Can you work these out from the model? Positions are in its coordinate system, mm. A direction names the side the tool comes from. Give positions to 0.01 mm unless a question says otherwise; leave off trailing zeros. Loops run counter-clockwise (first coordinate to the right, second up) from the corner with the lowest first, then second, coordinate; pieces in that order, holes last.
from build123d import *

# Parameters (mm, degrees)
SKETCH1_R           = 1.75
BOSS_EXTRUDE1_DEPTH = 5
SKETCH3_W           = 35
SKETCH3_H           = 20
SKETCH3_W_2         = 22.6
SKETCH3_H_2         = 12
BOSS_EXTRUDE4_DEPTH = 3
SKETCH6_W           = 15.399861764
SKETCH6_H           = 20
CUT_EXTRUDE2_DEPTH  = 76.166481892
SKETCH9_R           = 1
CUT_EXTRUDE4_DEPTH  = 7
SKETCH24_W          = 38
SKETCH24_H          = 25
BOSS_EXTRUDE8_DEPTH = 5
SKETCH27_R          = 2.3
CUT_EXTRUDE15_DEPTH = 4
FILLET9_R           = 4
SKETCH3_5_W         = 22.6
SKETCH3_5_H         = 12
CUT_EXTRUDE16_DEPTH = 3
BOSS_EXTRUDE9_DEPTH = 2
CUT_EXTRUDE18_DEPTH = 4
CUT_EXTRUDE19_DEPTH = 66.796921133
SKETCH37_W          = 38
SKETCH37_H          = 4.5
CUT_EXTRUDE20_DEPTH = 4


with BuildPart() as part:
    # Sketch1 → Boss-Extrude1 (new body)
    with BuildSketch(Plane(origin=(0, 0, 0), x_dir=(1, 0, 0), z_dir=(0, 1, 0))):
        Polygon((0, 33.819660113), (0, 15), (10, 0), (26, 0), (36, 15), (60, 15), (60, 35), (36, 35), (26, 45), (10, 45), align=None)
        with Locations(Location((13, 5, 0), (0, 0, 270))):
            Circle(SKETCH1_R, mode=Mode.SUBTRACT)
        with Locations(Location((23, 5, 0), (0, 0, 270))):
            Circle(SKETCH1_R, mode=Mode.SUBTRACT)
        with Locations(Location((5, 25, 0), (0, 0, 270))):
            Circle(SKETCH1_R, mode=Mode.SUBTRACT)
    extrude(amount=BOSS_EXTRUDE1_DEPTH)

    # Sketch3 → Boss-Extrude4 (add)
    with BuildSketch(Plane.XZ):
        with Locations((27.100138236, -25)):
            Rectangle(SKETCH3_W, SKETCH3_H)
        with Locations((27.100138236, -25)):
            Rectangle(SKETCH3_W_2, SKETCH3_H_2, mode=Mode.SUBTRACT)
    extrude(amount=BOSS_EXTRUDE4_DEPTH)

    # Sketch6 → Cut-Extrude2 (cut, through all)
    with BuildSketch(Plane.XZ):
        with Locations((52.300069118, -25)):
            Rectangle(SKETCH6_W, SKETCH6_H)
    extrude(amount=-CUT_EXTRUDE2_DEPTH, mode=Mode.SUBTRACT)

    # Sketch9 → Cut-Extrude4 (cut)
    with BuildSketch(Plane.XZ.offset(3)):
        with Locations((13.525138236, -25)):
            Circle(SKETCH9_R)
        with Locations((40.675138236, -25)):
            Circle(SKETCH9_R)
    extrude(amount=-CUT_EXTRUDE4_DEPTH, mode=Mode.SUBTRACT)

    # Sketch24 → Boss-Extrude8 (add)
    with BuildSketch(Plane(origin=(0, 0, -35), x_dir=(-1, 0, 0), z_dir=(0, 0, -1))):
        with Locations((-21.4, -0.25)):
            Rectangle(SKETCH24_W, SKETCH24_H)
    extrude(amount=BOSS_EXTRUDE8_DEPTH)

    # Sketch27 → Cut-Extrude15 (cut)
    with BuildSketch(Plane(origin=(0, 0, -40), x_dir=(-1, 0, 0), z_dir=(0, 0, -1))):
        with Locations((-21.4, -0.25)):
            Circle(SKETCH27_R)
    extrude(amount=-CUT_EXTRUDE15_DEPTH, mode=Mode.SUBTRACT)

    # Fillet9
    fillet9_edges = [part.edges().sort_by_distance(p)[0] for p in [
        (2.4, -12.75, -37.5),
        (40.4, 12.25, -37.5),
        (40.4, -12.75, -37.5),
        (2.4, 12.25, -37.5),
        (44.600138236, 1, -35),
        (44.600138236, 1, -15),
    ]]
    fillet(fillet9_edges, radius=FILLET9_R)

    # Sketch3_5 → Cut-Extrude16 (cut)
    with BuildSketch(Plane.XZ):
        with Locations((27.100138236, -25)):
            Rectangle(SKETCH3_5_W, SKETCH3_5_H)
    extrude(amount=-CUT_EXTRUDE16_DEPTH, mode=Mode.SUBTRACT)

    # Sketch34 → Boss-Extrude9 (add)
    with BuildSketch(Plane.XZ.offset(-3)):
        Polygon((38.400138236, -31), (44.400138238, -31), (44.400138238, -25), (44.400138238, -19), (38.400138236, -19), (15.800138236, -19), (15.800138236, -31), align=None)
    extrude(amount=BOSS_EXTRUDE9_DEPTH)

    # Sketch35 → Cut-Extrude18 (cut)
    with BuildSketch(Plane.XZ.offset(-1)):
        with BuildLine():
            Line((26.100324519, -22.482250986), (26.945782176, -22.499999995))
            ThreePointArc((26.945782176, -22.499999995), (38.400138236, -25), (26.945782176, -27.500000005))
            Line((26.945782176, -27.500000005), (26.100324492, -27.482252247))
            ThreePointArc((26.100324492, -27.482252247), (23.600323888, -24.982251603), (26.100324519, -22.482250986))
        make_face()
    extrude(amount=-CUT_EXTRUDE18_DEPTH, mode=Mode.SUBTRACT)

    # Sketch36 → Cut-Extrude19 (cut, through all)
    with BuildSketch(Plane(origin=(0, 5, 0), x_dir=(1, 0, 0), z_dir=(0, 1, 0))):
        Polygon((5.527864045, 40), (31, 40), (26, 45), (10, 45), align=None)
    extrude(amount=-CUT_EXTRUDE19_DEPTH, mode=Mode.SUBTRACT)

    # Sketch37 → Cut-Extrude20 (cut)
    with BuildSketch(Plane.XY.offset(-35)):
        with Locations((21.4, 7.25)):
            Rectangle(SKETCH37_W, SKETCH37_H)
    extrude(amount=-CUT_EXTRUDE20_DEPTH, mode=Mode.SUBTRACT)


solid = part.part
(1) Thinking about a two-plate mould opening in Z: for faces 1 (the flat face through (21, 9.5, -37)), 2 (the flat face through (14, 4, -25)), 3 (the flat face through (22, 11, -35)), which applies, pulls with the +Z half, pulls with the -Z half, needs draft (parallel to the pull), parting line crosses it, or undercut?
Returned:
face 1: needs draft
face 2: undercut
face 3: pulls with the +Z half
(2) Suppose I cut it at D-D on z = -9. List the corners of the cut face in (x, y) for me, plus the area to 3 significant figures.
Returned:
outline: (4, 0) - (32, 0) - (32, 5) - (4, 5) - close
area: 140 mm2
(3) Suppose I cut it at C-C on y = 6. List the corners of the cut face in (x, z) for me.
Returned:
outline: (2.4, -40) - (40.4, -40) - (40.4, -39) - (2.4, -39) - close
(4) Please list where these lines run through material, in increasing order: probe 1 along Z at (x, y) = (13.5, 0.75); probe 2 along Y at (x, z) = (28, -38); probe 3 along Y at (x, z) = (35.5, -16).
Returned:
probe 1: z = -40 to -26, -24 to -6.68, -3.32 to 0
probe 2: y = -12.75 to 5, 9.5 to 12.25
probe 3: y = -3 to 5
(5) Suppose I cut it at B-B on x = 23. List the corners of the cut face in (y, z) for me, plus the area to 3 significant figures.
Returned:
outline: (-12.75, -40) - (-1.9, -40) - (-1.9, -36) - (1.4, -36) - (1.4, -40) - (12.25, -40) - (12.25, -35) - (9.5, -35) - (9.5, -39) - (5, -39) - (5, -6.75) - (0, -6.75) - (0, -15) - (-3, -15) - (-3, -19) - (1, -19) - (1, -31) - (-3, -31) - (-3, -35) - (-12.75, -35) - close; (0, -3.25) - (5, -3.25) - (5, 0) - (0, 0) - close
area: 263 mm2
(6) Which directions (+Z, -Z, +X, -X, +Y, -Y) give clear straight access to the entire face, cutting with the end or side of a thin tool? Please do faces 4 (the cylindrical face through (19.206, 0.441, -38.028)), 5 (the flat face through (41, 4, -25)), 6 (the flat face through (2.4, -2, -38)), 7 (the cylindrical face through (40.458, -1.028, -25.976)).
Returned:
face 4: -Z
face 5: none
face 6: -Z, -X, -Y
face 7: -Y
(7) Suppose I cut it at A-A on z = -5. List the corners of the cut face in (x, y) for me, plus the area to 3 significant figures.
Returned:
outline: (6.67, 0) - (11.25, 0) - (11.25, 5) - (6.67, 5) - close; (14.75, 0) - (21.25, 0) - (21.25, 5) - (14.75, 5) - close; (24.75, 0) - (29.33, 0) - (29.33, 5) - (24.75, 5) - close
area: 78.3 mm2
(8) Will these pins go through, and if not, where does the flat tip stop? P1, Ø2, axis at x = 6.5, y = -3.5, coming from the +Z side; P2, Ø2, axis at x = 13, z = -5, coming from the -Y side; P3, Ø8, axis at y = 3, z = -7, coming from the -X side; P4, Ø6, axis at y = 7.5, z = -10.5, coming from the +X side.
Returned:
P1: stops at z = -35
P2: passes through
P3: stops at x = 2.67
P4: stops at x = 34.11
